```python
from build123d import *

# Parameters (mm, degrees)
ESBO_O1_R                  = 60.802005659
ESBO_O1_R_2                = 54.579770148
RESSALTO_EXTRUS_O1_DEPTH   = 100
ESBO_O1_R_3                = 33.324434684
ESBO_O1_R_4                = 14.070831149
RESSALTO_EXTRUS_O1_2_DEPTH = 100
ESBO_O3_R                  = 14.070831149
RESSALTO_EXTRUS_O2_DEPTH   = 10
ESBO_O1_3_R                = 54.579770148
ESBO_O1_3_R_2              = 33.324434684
RESSALTO_EXTRUS_O3_DEPTH   = 10


with BuildPart() as part:
    # Esbo_o1 → Ressalto-extrus_o1 (new body)
    with BuildSketch(Plane(origin=(0, 0, 0), x_dir=(1, 0, 0), z_dir=(0, 1, 0))):
        with Locations(Location((0, 0, 0), (0, 0, 270))):
            Circle(ESBO_O1_R)
        with Locations(Location((0, 0, 0), (0, 0, 270))):
            Circle(ESBO_O1_R_2, mode=Mode.SUBTRACT)
    extrude(amount=RESSALTO_EXTRUS_O1_DEPTH)



with BuildPart() as body_2:
    # Esbo_o1 → Ressalto-extrus_o1 2 (new body)
    with BuildSketch(Plane(origin=(0, 0, 0), x_dir=(1, 0, 0), z_dir=(0, 1, 0))):
        with Locations(Location((0, 0, 0), (0, 0, 270))):
            Circle(ESBO_O1_R_3)
        with Locations(Location((0, 0, 0), (0, 0, 270))):
            Circle(ESBO_O1_R_4, mode=Mode.SUBTRACT)
    extrude(amount=RESSALTO_EXTRUS_O1_2_DEPTH)

    # Esbo_o3 → Ressalto-extrus_o2 (add)
    with BuildSketch(Plane(origin=(0, 100, 0), x_dir=(1, 0, 0), z_dir=(0, 1, 0))):
        with Locations(Location((0, 0, 0), (0, 0, 270))):
            Circle(ESBO_O3_R)
    extrude(amount=-RESSALTO_EXTRUS_O2_DEPTH)


with BuildPart() as part_1:
    add(part.part)

    add(body_2.part)  # Ressalto-extrus_o3 merges body 2
    # Esbo_o1_3 → Ressalto-extrus_o3 (add)
    with BuildSketch(Plane(origin=(0, 0, 0), x_dir=(1, 0, 0), z_dir=(0, 1, 0))):
        with Locations(Location((0, 0, 0), (0, 0, 270))):
            Circle(ESBO_O1_3_R)
        with Locations(Location((0, 0, 0), (0, 0, 270))):
            Circle(ESBO_O1_3_R_2, mode=Mode.SUBTRACT)
    extrude(amount=RESSALTO_EXTRUS_O3_DEPTH)


solid = part_1.part
```
Input: part model. Units: mm. Frame: model coordinates. A direction names the side the tool comes from. Coordinates: 2 decimals unless noted, no trailing zeros. Loops run counter-clockwise (first coordinate to the right, second up) from the corner with the lowest first, then second, coordinate; pieces in that order, holes last. Notation, with made-up numbers: (34.25, 17.5) -> (79.25, 17.5) arc R25 ccw to (79.25, 35.5) -> close; hole circle Ø3 at (26, -39.5). An arc over 180 degrees is marked (long way). Use a Markdown table: item, result.
1) Cut plane B-B (x = 0). Return the cut outline in (y, z).
Results found:
| item | result |
|---|---|
| outline | (0, -60.8) -> (100, -60.8) -> (100, -54.58) -> (10, -54.58) -> (10, -33.32) -> (100, -33.32) -> (100, 33.32) -> (10, 33.32) -> (10, 54.58) -> (100, 54.58) -> (100, 60.8) -> (0, 60.8) -> (0, 14.07) -> (90, 14.07) -> (90, -14.07) -> (0, -14.07) -> close |
2) Access query for faces 5 (the cylindrical face through (-53.282, 54.37, -11.832)), 6 (the flat face through (14.4, 0, -0.9)). Directions: +Z, -Z, +X, -X, +Y, -Y. A direction counts if a zero-diameter tool reaches every point of the face in a straight line with its end or side. Return the directions, or none.
Results found:
| item | result |
|---|---|
| face 5 | +Y |
| face 6 | +Z, -Z, +X, -X, -Y |
3) Cut plane D-D (y = 93). Return the cut outline in (x, z).
Results found:
| item | result |
|---|---|
| outline | circle Ø121.6 at (0, 0); circle Ø66.65 at (0, 0); hole circle Ø109.16 at (0, 0) |
4) Cut plane A-A (y = 43). Return the cut outline in (x, z).
Results found:
| item | result |
|---|---|
| outline | circle Ø121.6 at (0, 0); circle Ø66.65 at (0, 0); hole circle Ø109.16 at (0, 0); hole circle Ø28.14 at (0, 0) |
5) Contact query for flat-ended pins moving along their axis: pin 1 (8.5 mm diameter, centred on x = 5, z = -4, fed in from -Y); pin 2 (4 mm diameter, centred on x = -31.5, y = 51, fed in from +Z); pin 3 (1.5 mm diameter, centred on x = -29.5, z = 41.5, fed in from +Y). Output: stop coordinate, or through.
Results found:
| item | result |
|---|---|
| pin 1 | stops at y = 90 |
| pin 2 | stops at z = 53.17 |
| pin 3 | stops at y = 10 |
6) Cut plane C-C (z = 0). Return the cut outline in (x, y), then the cut area to 3 significant figures.
Results found:
| item | result |
|---|---|
| outline | (-60.8, 0) -> (-14.07, 0) -> (-14.07, 90) -> (14.07, 90) -> (14.07, 0) -> (60.8, 0) -> (60.8, 100) -> (54.58, 100) -> (54.58, 10) -> (33.32, 10) -> (33.32, 100) -> (-33.32, 100) -> (-33.32, 10) -> (-54.58, 10) -> (-54.58, 100) -> (-60.8, 100) -> close |
| area | 5,800 mm2 |
7) Material intervals for line 1 along X through (y, z) = (69, 0); line 2 along X through (y, z) = (72, 1); line 3 along X through (y, z) = (21.5, 29), sorted ascending. Write a range as from..to.
Results found:
| item | result |
|---|---|
| line 1 | x = -60.8..-54.58, -33.32..-14.07, 14.07..33.32, 54.58..60.8 |
| line 2 | x = -60.79..-54.57, -33.31..-14.04, 14.04..33.31, 54.57..60.79 |
| line 3 | x = -53.44..-46.24, -16.42..16.42, 46.24..53.44 |
8) Pull-direction query (X, two-part tool) for faces 1 (the flat face through (23, 100, -50)), 2 (the cylindrical face through (-8.56, 44.37, -11.17)), 3 (the cylindrical face through (-37, 49.3, -48.25)), 4 (the flat face through (0, 90, 0)); classes: released by +X, released by -X, zero draft, split by the parting line, or undercut.
Results found:
| item | result |
|---|---|
| face 1 | zero draft |
| face 2 | undercut |
| face 3 | split by the parting line |
| face 4 | undercut |
